Read the model definition and answer for the solid it produces. Units are mm, in the model's axes. Give positions to 0.01 mm unless a question says otherwise; leave off trailing zeros. Order: outer loops, then holes, each group sorted by start corner. A loop starts at its lowest first (then second) coordinate and runs counter-clockwise, first axis right, second up. Notation, with made-up numbers: (72, 32.5) - (114, 32.5) arc R14 ccw to (114, 54.5) - close; hole circle Ø4 at (-9, 81). An arc over 180 degrees is marked (long way). Write each question's results on one line, items separated by ' | '. Start each with the question number.
Q1. Find section A-A on z = 856.5. Give the vertices of the cut face in (x, y), and give its area (3 significant figures).
Q2. Find section B-B on y = -15.75. Give the vertices of the cut face in (x, z), and give its area (3 significant figures).
Q3. Find the intervals of material crossed by line 1 along X through (y, z) = (-14.75, 661); line 2 along Z through (x, y) = (17, -5.5); line 3 along Y through (x, z) = (22, 1539), in increasing order. Write a range as from..to.
Q4. Flat-ended cylindrical pins translate along their axes: P1, Ø10.5, axis at x = 27.5, z = 1021.5, coming from the -Y side; P2, Ø8, axis at x = 27, y = -13, coming from the +Z side; P3, Ø10, axis at x = -55, y = -11.5, coming from the +Z side. Find the tip coordinate at first contact, or state that the pin passes through.
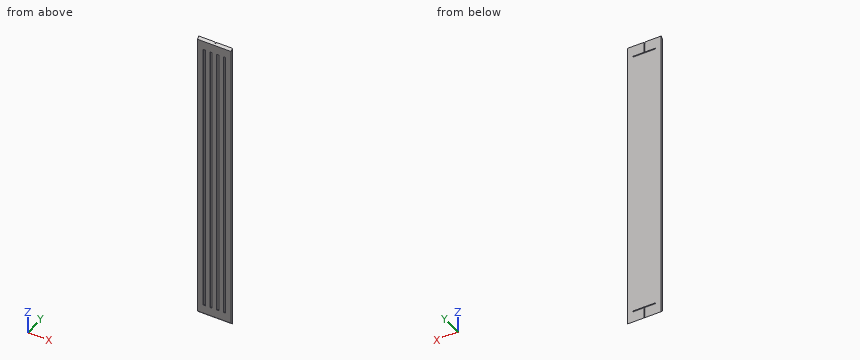
from build123d import *

# Parameters (mm, degrees)
F0_W     = 304.8
F0_H     = 2628.9
F1_DEPTH = 19.05
F2_SIZE  = 19.04999
F3_W     = 21.082
F3_H     = 2438.4
F4_DEPTH = 10.16
F5_W     = 9.525
F5_H     = 95.25
F6_DEPTH = 6.35


# Not quite as in the source:
# - a fillet or chamfer is up to 0.001 mm smaller than in the source, because OpenCascade refuses the exact size


with BuildPart() as f1:
    # F0 (on Front) → F1 (new body)
    with BuildSketch(Plane.XZ):
        with Locations((-2.8532538563, 1186.9243339048)):
            Rectangle(F0_W, F0_H)
    extrude(amount=F1_DEPTH)

    # F2 (size 19.05 in the source; OpenCascade refuses exactly that, so slightly less here)
    f2_edges = [f1.edges().sort_by_distance(p)[0] for p in [
        (-2.853254, -19.05, 2501.374334),
        (-2.853254, -19.05, -127.525666),
    ]]
    chamfer(f2_edges, length=F2_SIZE)

    # F3 (on face) → F4 (cut)
    with BuildSketch(Plane.XZ.offset(19.05)):
        with Locations((-94.2932538563, 1186.9243339048)):
            Rectangle(F3_W, F3_H)
        with Locations((-33.3332538563, 1186.9243339048)):
            Rectangle(F3_W, F3_H)
        with Locations((27.6267461437, 1186.9243339048)):
            Rectangle(F3_W, F3_H)
        with Locations((88.5867461437, 1186.9243339048)):
            Rectangle(F3_W, F3_H)
    extrude(amount=-F4_DEPTH, mode=Mode.SUBTRACT)

    # F5 (on face) → F6 (cut)
    with BuildSketch(Plane(origin=(0, 0, 0), x_dir=(-1, 0, 0), z_dir=(0, 1, 0))):
        Polygon((-1.9092461437, 2406.1243339048), (-99.1277461437, 2406.1243339048), (-99.1277461437, 2396.5993339048), (104.8342538563, 2396.5993339048), (104.8342538563, 2406.1243339048), (7.6157538563, 2406.1243339048), align=None)
        with Locations((2.8532538563, 2453.7493339048)):
            Rectangle(F5_W, F5_H)
        with Locations((2.8532538563, -79.9006660952)):
            Rectangle(F5_W, F5_H)
        Polygon((-99.1277461437, -32.2756660952), (-1.9092461437, -32.2756660952), (7.6157538563, -32.2756660952), (104.8342538563, -32.2756660952), (104.8342538563, -22.7506660952), (-99.1277461437, -22.7506660952), align=None)
    extrude(amount=-F6_DEPTH, mode=Mode.SUBTRACT)


solid = f1.part
Working result:
1) outline: (-155.25, -19.05) - (-104.83, -19.05) - (-104.83, -8.89) - (-83.75, -8.89) - (-83.75, -19.05) - (-43.87, -19.05) - (-43.87, -8.89) - (-22.79, -8.89) - (-22.79, -19.05) - (17.09, -19.05) - (17.09, -8.89) - (38.17, -8.89) - (38.17, -19.05) - (78.05, -19.05) - (78.05, -8.89) - (99.13, -8.89) - (99.13, -19.05) - (149.55, -19.05) - (149.55, 0) - (-155.25, 0) - close | area: 4,950 mm²
2) outline: (-155.25, -111.78) - (149.55, -111.78) - (149.55, 2485.62) - (-155.25, 2485.62) - close; hole (-104.83, -32.28) - (-83.75, -32.28) - (-83.75, 2406.12) - (-104.83, 2406.12) - close; hole (-43.87, -32.28) - (-22.79, -32.28) - (-22.79, 2406.12) - (-43.87, 2406.12) - close; hole (17.09, -32.28) - (38.17, -32.28) - (38.17, 2406.12) - (17.09, 2406.12) - close; hole (78.05, -32.28) - (99.13, -32.28) - (99.13, 2406.12) - (78.05, 2406.12) - close | area: 586,000 mm²
3) line 1: -155.25..-104.83, -83.75..-43.87, -22.79..17.09, 38.17..78.05, 99.13..149.55 | line 2: -122.03..-32.28, -22.75..2396.6, 2406.12..2495.87 | line 3: -8.89..0
4) P1: y = -8.89 | P2: z = 2492.37 | P3: z = 2494.87
